from build123d import *

# Parameters (mm, degrees)
F1_DEPTH = 152.4
F3_DEPTH = 17.526


with BuildPart() as f1:
    # F0 (on Front) → F1 (new body, symmetric)
    with BuildSketch(Plane.XZ):
        with BuildLine():
            Line((-0.476688, -84.644368), (0, -85.725))
            ThreePointArc((0, -85.725), (55.88, 0), (0, 85.725))
            Line((0, 85.725), (-0.476688, 84.644368))
            ThreePointArc((-0.476688, 84.644368), (54.6989, 0), (-0.476688, -84.644368))
        make_face()
    extrude(amount=F1_DEPTH, both=True)

    # F2 (on face) → F3 (join)
    with BuildSketch(Plane.XZ.offset(152.4)):
        with BuildLine():
            Line((-0.476688, 84.644368), (-0.476688, -84.644368))
            ThreePointArc((-0.476688, -84.644368), (54.6989, 0), (-0.476688, 84.644368))
        make_face()
    extrude(amount=-F3_DEPTH)

    # F4: F1 across plane


with BuildPart() as f1_1:
    add(f1.part)
    add(f1.part.mirror(Plane.XZ))


solid = f1_1.part
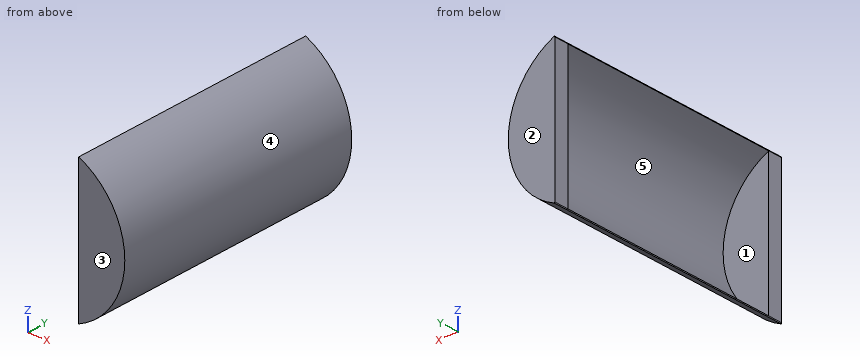
Verification items for the finished model (mm, model axes). Face numbers are marked on the shaded views. A direction names the side the tool comes from. Give positions to 0.01 mm unless a question says otherwise; leave off trailing zeros. Loops run counter-clockwise (first coordinate to the right, second up) from the corner with the lowest first, then second, coordinate; pieces in that order, holes last.
1) Thickness scan on line 1 along Y through (x, z) = (9, -17.5); line 2 along Z through (x, y) = (44, -78.5); line 3 along Z through (x, y) = (41, -69.5). Record the ranges inside material, lowest first.
2) Sectioned sample at A-A, the plane x = 15.5. Enter the section's corners in (y, z), then the cut area to 3 significant figures.
3) Draft check along Y on the marked faces 3, 4 and 5. Enter one of: pulls with the +Y half, pulls with the -Y half, needs draft (parallel to the pull), parting line crosses it, or undercut.
4) Sectioned sample at B-B, the plane z = 7. Enter the section's corners in (x, y), then the cut area to 3 significant figures.
5) Sectioned sample at D-D, the plane x = 40. Enter the section's corners in (y, z), then the cut area to 3 significant figures.
6) Sectioned sample at C-C, the plane y = -39.5. Enter the section's corners in (x, z) (3 decimals).
7) Depth check by flat-ended pin: pin 1 Ø2 at (y, z) = (53, -28.5) entering from +X; pin 2 Ø3 at (x, y) = (7, 49) entering from -Z; pin 3 Ø12 at (y, z) = (82.5, -41) entering from +X. Enter the tip coordinate at first touch or a pass-through.
8) Set-up check for the marked faces 1 and 2: record each of +Z, -Z, +X, -X, +Y, -Y from which the full face is reachable in a straight line by a thin tool's end or side.
Answers:
1. line 1: y = -152.4 to -134.87, 134.87 to 152.4
1. line 2: z = -45.66 to -43.19, 43.19 to 45.66
1. line 3: z = -50.67 to -48.45, 48.45 to 50.67
2. outline: (-152.4, -77.05) - (152.4, -77.05) - (152.4, 77.05) - (-152.4, 77.05) - close; hole (-134.87, -75.61) - (134.87, -75.61) - (134.87, 75.61) - (-134.87, 75.61) - close
2. area: 6,180 mm2
3. face 3: pulls with the -Y half
3. face 4: needs draft
3. face 5: undercut
4. outline: (-0.48, -152.4) - (55.62, -152.4) - (55.62, 152.4) - (-0.48, 152.4) - (-0.48, 134.87) - (54.43, 134.87) - (54.43, -134.87) - (-0.48, -134.87) - close
4. area: 2,290 mm2
5. outline: (-152.4, -52.19) - (152.4, -52.19) - (152.4, 52.19) - (-152.4, 52.19) - close; hole (-134.87, -50.04) - (134.87, -50.04) - (134.87, 50.04) - (-134.87, 50.04) - close
5. area: 4,820 mm2
6. outline: (-0.477, -84.644) - (0, -85.725) arc R93.695 ccw to (0, 85.725) - (-0.477, 84.644) arc R92.514 cw to start
7. pin 1: stops at x = 51.75
7. pin 2: stops at z = -83.08
7. pin 3: stops at x = 49.1
8. face 1: -X
8. face 2: +Z, -Z, +X, -X, +Y
